Work out the finished part from the listing and answer in its coordinate system (mm). Give positions to 0.01 mm unless a question says otherwise; leave off trailing zeros. Order: outer loops, then holes, each group sorted by start corner. A loop starts at its lowest first (then second) coordinate and runs counter-clockwise, first axis right, second up. Notation, with made-up numbers: (20.5, 27) - (37.5, 27) arc R23 cw to (37.5, 57) - close; hole circle Ø7 at (54.5, 30.5). An arc over 180 degrees is marked (long way). Write each question's results on one line, items separated by ' | '.
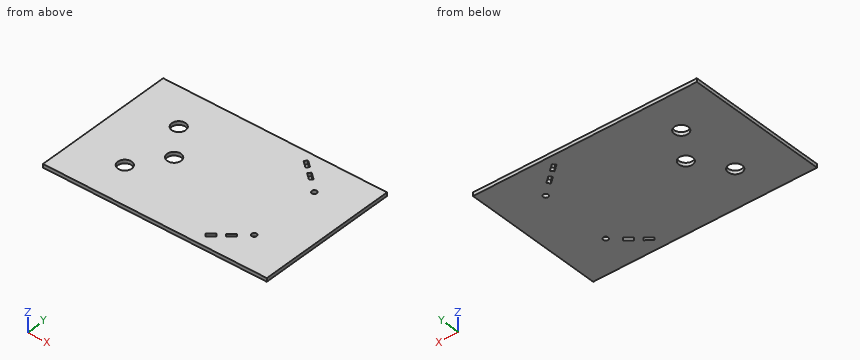
from build123d import *

# Parameters (mm, degrees)
SKETCH1_W           = 400.05
SKETCH1_H           = 254
BOSS_EXTRUDE1_DEPTH = 6.35
SKETCH2_R           = 4.5
SKETCH2_R_2         = 12.446
CUT_EXTRUDE1_DEPTH  = 6.35


with BuildPart() as part:
    # Sketch1 → Boss-Extrude1 (new body)
    with BuildSketch(Plane.XY):
        with Locations((200.025, 127)):
            Rectangle(SKETCH1_W, SKETCH1_H)
    extrude(amount=BOSS_EXTRUDE1_DEPTH)

    # Sketch2 → Cut-Extrude1 (cut)
    with BuildSketch(Plane.XY.offset(6.35)):
        with Locations((323.85, 63.5)):
            Circle(SKETCH2_R)
        with Locations((323.85, 190.5)):
            Circle(SKETCH2_R)
        with Locations((127, 127)):
            Circle(SKETCH2_R_2)
        with Locations((87, 70)):
            Circle(SKETCH2_R_2)
        with Locations((87, 184)):
            Circle(SKETCH2_R_2)
        Polygon((275.320145198, 17.766787665), (287.027837499, 27.523197916), (282.962666561, 32.401403041), (271.25497426, 22.64499279), align=None)
        Polygon((296.78424775, 35.653539792), (308.491940051, 45.409950042), (304.426769113, 50.288155168), (292.719076812, 40.531744917), align=None)
        Polygon((271.25497426, 239.620854783), (282.962666561, 229.864444532), (278.897495623, 224.986239407), (267.189803322, 234.742649658), align=None)
        Polygon((292.719076812, 221.734102657), (304.426769113, 211.977692406), (300.361598175, 207.09948728), (288.653905874, 216.855897531), align=None)
    extrude(amount=-CUT_EXTRUDE1_DEPTH, mode=Mode.SUBTRACT)


solid = part.part
1. A cutting plane is placed at D-D, the plane y = 190.5. Write down the section's boundary in (x, z), then the cut area to 3 significant figures.
Answer list:
outline: (0, 0) - (76.39, 0) - (76.39, 6.35) - (0, 6.35) - close; (97.61, 0) - (319.35, 0) - (319.35, 6.35) - (97.61, 6.35) - close; (328.35, 0) - (400.05, 0) - (400.05, 6.35) - (328.35, 6.35) - close | area: 2,350 mm^2
2. Straight lines are drawn through the part: line 1 (Y direction, x = 87, z = 3); line 2 (Y direction, x = 323.85, z = 2.25); line 3 (X direction, y = 216.5, z = 5.5). For each, find the intervals that lie inside material, in ascending order. Write a range as [from, to].
Answer list:
line 1: [0, 57.55], [82.45, 171.55], [196.45, 254] | line 2: [0, 59], [68, 186], [195, 254] | line 3: [0, 289.08], [299, 400.05]
3. A cutting plane is placed at B-B, the plane x = 323.85. Write down the section's boundary in (y, z), then the cut area to 3 significant figures.
Answer list:
outline: (0, 0) - (59, 0) - (59, 6.35) - (0, 6.35) - close; (68, 0) - (186, 0) - (186, 6.35) - (68, 6.35) - close; (195, 0) - (254, 0) - (254, 6.35) - (195, 6.35) - close | area: 1,500 mm^2
4. A cutting plane is placed at A-A, the plane x = 127. Write down the section's boundary in (y, z).
Answer list:
outline: (0, 0) - (114.55, 0) - (114.55, 6.35) - (0, 6.35) - close; (139.45, 0) - (254, 0) - (254, 6.35) - (139.45, 6.35) - close
5. A cutting plane is placed at C-C, the plane z = 2.25. State how many separate pieces and enclosed holes the cut face has, then the cut area to 3 significant figures.
Answer list:
separate pieces: 1 | enclosed holes: 9 | area: 99,600 mm^2
